The listing builds one solid part. Answer for the finished solid, in the listing's coordinates (mm). Face numbers are marked on the shaded views. Give positions to 0.01 mm unless a question says otherwise; leave off trailing zeros. Loops run counter-clockwise (first coordinate to the right, second up) from the corner with the lowest first, then second, coordinate; pieces in that order, holes last. Notation, with made-up numbers: M -2,-1.5 L 26,-1.5 A15 ccw 26,15.5 Z; hole C -31,25.25 d10. An arc over 180 degrees is marked long. Use one line per item in the form item = value. Start each with the question number.
1. The part is cut by section D-D (y = 1.3). Write down the section's boundary in (x, z).
2. Each of these flat-tipped pins is pushed along its axis until it touches: pin 1 Ø1 at (x, y) = (-5, 1.5) entering from +Z; pin 2 Ø1 at (y, z) = (1, -3) entering from -X; pin 3 Ø1 at (x, y) = (0, 3.5) entering from +Z. Where does it stop, or does it pass through?
3. The mould has two halves that part along Z. Classify the marked faces 1 and 2: released by +Z, released by -Z, zero draft, split by the parting line, or undercut.
4. The part is cut by section C-C (y = 2.7). Write down the section's boundary in (x, z).
5. Straight lines are drawn through the part: line 1 (Z direction, x = 0, y = 3.7); line 2 (X direction, y = 3.3, z = 0). For each, find the intervals that lie inside material, in ascending order. Write a range as from..to.
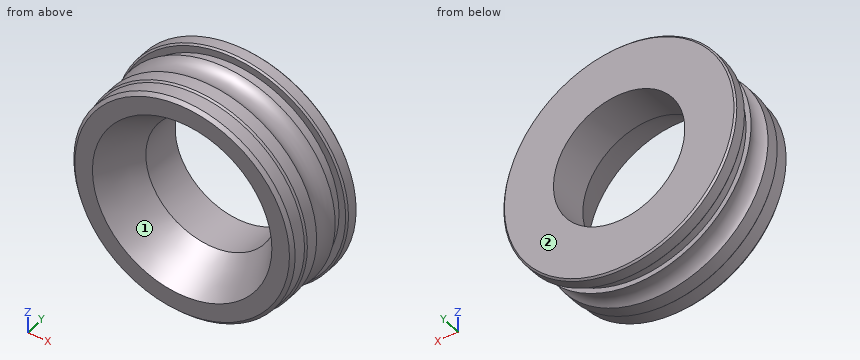
from build123d import *


with BuildPart() as part:
    # Croquis1 → Revolución1 (revolve)
    with BuildSketch(Plane.XY):
        with BuildLine():
            Line((6.45, 0), (6.65, 0.2))
            Line((6.65, 0.2), (6.65, 1))
            Line((6.65, 1), (6.75, 1.1))
            Line((6.75, 1.1), (6.75, 1.767))
            Line((6.75, 1.767), (6.75, 1.889))
            ThreePointArc((6.75, 1.889), (6.429860393, 2.6559209), (6.8, 3.4))
            Line((6.8, 3.4), (6.5, 3.4))
            Line((6.5, 3.4), (6.5, 4.15))
            Line((6.5, 4.15), (6.9, 4.15))
            Line((6.9, 4.15), (7, 4.25))
            Line((7, 4.25), (7, 4.9))
            Line((7, 4.9), (6.9, 5))
            Line((6.9, 5), (3.95, 5))
            Line((3.95, 5), (3.95, 2.5))
            Line((3.95, 2.5), (5.393375673, 0))
            Line((5.393375673, 0), (6.45, 0))
        make_face()
    revolve(axis=Axis((0, 0, 0), (0, 1, 0)))


solid = part.part
Derived:
q1.outline = C 0,0 d13.5; hole C 0,0 d9.29
q2.pin_1 = 5.03
q2.pin_2 = -6.27
q2.pin_3 = 6.8
q3.face_1 = undercut
q3.face_2 = zero draft
q4.outline = C 0,0 d12.86; hole C 0,0 d7.9
q5.line_1 = -6.5..-3.95, 3.95..6.5
q5.line_2 = -6.69..-3.95, 3.95..6.69
